Can you work these out from the drawing? Everything is in mm from the part's minimum corner. A direction names the side the tool comes from. Round coordinates to 2 decimals unless told otherwise and drop trailing zeros. Order: outer loops, then holes, each group sorted by start corner. A loop starts at its lowest first (then second) coordinate and runs counter-clockwise, first axis right, second up. Notation, with made-up numbers: (58.5, 56) -> (111.5, 56) arc R24 cw to (111.5, 73) -> close; hole circle Ø9 at (1.5, 65). An arc over 180 degrees is marked (long way). One line per item, written item: value.
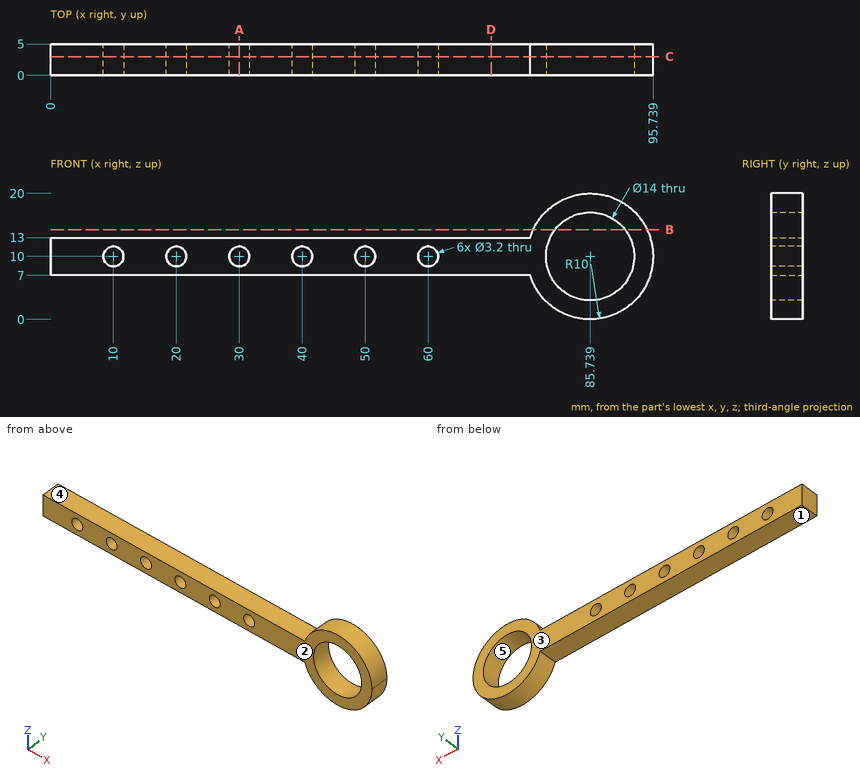
Q1. I want a section at B-B on z = 14.25. List the corners of the cut face in (x, y) for me.
Answers below:
outline: (76.69, 0) -> (80.18, 0) -> (80.18, 5) -> (76.69, 5) -> close; (91.3, 0) -> (94.79, 0) -> (94.79, 5) -> (91.3, 5) -> close
Q2. I want a section at D-D on x = 70. List the corners of the cut face in (y, z) for me.
Answers below:
outline: (0, 7) -> (5, 7) -> (5, 13) -> (0, 13) -> close
Q3. On a 3-axis mill with a long thin cutter (end or side, diameter ignored), from which of +Z, -Z, +X, -X, +Y, -Y can I reach the whole of each face in a straight line? I mean the marked faces 1 and 2. Say none if no direction works.
Answers below:
face 1: -Z, -X, +Y, -Y
face 2: +Z, -Z, +X, -X, -Y
Q4. Will these pins go through, and if not, where does the flat tip stop? pin 1 Ø2.5 at (x, y) = (41, 3.5) entering from -Z; pin 2 Ø1 at (y, z) = (2, 9) entering from +X; pin 3 Ø1.5 at (y, z) = (1, 5) entering from -X; pin 4 Ø1.9 at (x, z) = (60, 10) entering from -Y.
Answers below:
pin 1: z = 7
pin 2: x = 95.73
pin 3: x = 76.69
pin 4: through
Q5. I want a section at C-C on y = 3. List the corners of the cut face in (x, z) for me.
Answers below:
outline: (0, 7) -> (76.2, 7) arc R10 ccw (long way) to (76.2, 13) -> (0, 13) -> close; hole circle Ø3.2 at (10, 10); hole circle Ø3.2 at (20, 10); hole circle Ø3.2 at (30, 10); hole circle Ø3.2 at (40, 10); hole circle Ø3.2 at (50, 10); hole circle Ø3.2 at (60, 10); hole circle Ø14 at (85.74, 10)
Q6. Please list where these lines run through material, in increasing order: line 1 along Z through (x, y) = (20, 1.15); line 2 along Z through (x, y) = (34, 1.85); line 3 along X through (y, z) = (4.1, 7.5).
Answers below:
line 1: 7 to 8.4, 11.6 to 13
line 2: 7 to 13
line 3: 0 to 79.2, 92.28 to 95.42
Q7. I want a section at A-A on x = 30. List the corners of the cut face in (y, z) for me.
Answers below:
outline: (0, 7) -> (5, 7) -> (5, 8.4) -> (0, 8.4) -> close; (0, 11.6) -> (5, 11.6) -> (5, 13) -> (0, 13) -> close
Q8. We'd pull the mould along Z, two halves only. Please class the marked faces 3, 4 and 5: released by +Z, released by -Z, zero draft, split by the parting line, or undercut.
Answers below:
face 3: zero draft
face 4: released by +Z
face 5: undercut
